Input: part model. Units: mm. Frame: model coordinates. A direction names the side the tool comes from. Round coordinates to 2 decimals unless told otherwise and drop trailing zeros. Loops run counter-clockwise (first coordinate to the right, second up) from the corner with the lowest first, then second, coordinate; pieces in that order, holes last. Notation, with made-up numbers: M -16.75,-3 L 31.25,-3 A19 ccw 31.25,16 Z; hole C 11,-28.5 d3. An arc over 180 degrees is marked long. Return JSON: item names as keys, results as strings. Group by question number.
1) Section D-D (z = 24). Output: boundary loops of the cut face in (x, y), plus the area to 3 significant figures.
2) Mould query, pull axis X, two halves, no side actions, for faces 1 (the face through (-34.962, 11.959, -7.764)), 2 (the face through (-7.5, 0, -8.5)), 3 (the face through (-3.3, 3.73, 10.48)). Classes: +X half, -X half, draft (parallel to the pull), parting line (faces both ways), or undercut.
3) Section A-A (z = 0). Output: boundary loops of the cut face in (x, y).
4) Section B-B (x = 0). Output: boundary loops of the cut face in (y, z), plus the area to 3 significant figures.
5) Section C-C (y = 11.5). Output: boundary loops of the cut face in (x, z).
6) Access query for faces 4 (the face through (3.3, 20.63, 10.48)), 5 (the face through (-9.21, 12.2, -2.05)), 6 (the face through (-9, 7.353, -3.31)). Directions: +Z, -Z, +X, -X, +Y, -Y. A direction counts if a zero-diameter tool reaches every point of the face in a straight line with its end or side. Return the directions, or none.
7) Contact query for flat-ended pins moving along their axis: P1, Ø12, axis at y = 18, z = 11.5, coming from the +X side; P2, Ø10, axis at x = 19.5, y = 19, coming from the +Z side; P3, Ø10, axis at y = 19, z = -13.5, coming from the +X side; P4, Ø13, axis at x = 0, z = 0, coming from the -Y side. Output: stop coordinate, or through.
8) Material intervals for line 1 (X direction, y = 3.5, z = 0); line 2 (X direction, y = 13.25, z = 0); line 3 (Z direction, x = -2.5, y = 15), sorted ascending. Write a range as from..to.
from build123d import *

# Parameters (mm, degrees)
SKETCH1_R           = 35.814
BOSS_EXTRUDE1_DEPTH = 24.257
SKETCH2_R           = 9.4361
CUT_EXTRUDE1_DEPTH  = 57.157699748
SKETCH3_R           = 10.9855
CUT_EXTRUDE2_DEPTH  = 7.3533
CUT_EXTRUDE3_START  = -7.3533
SKETCH4_R           = 10.9855
CUT_EXTRUDE3_DEPTH  = 7.3533


with BuildPart() as part:
    # Sketch1 → Boss-Extrude1 (new body)
    with BuildSketch(Plane(origin=(0, 0, 0), x_dir=(1, 0, 0), z_dir=(0, 1, 0))):
        with Locations(Location((0, 0, 0), (0, 0, 270))):
            Circle(SKETCH1_R)
    extrude(amount=BOSS_EXTRUDE1_DEPTH)

    # Sketch2 → Cut-Extrude1 (cut, through all)
    with BuildSketch(Plane(origin=(0, 24.257, 0), x_dir=(1, 0, 0), z_dir=(0, 1, 0))):
        with Locations(Location((0, 0, 0), (0, 0, 270))):
            Circle(SKETCH2_R)
    extrude(amount=-CUT_EXTRUDE1_DEPTH, mode=Mode.SUBTRACT)

    # Sketch3 → Cut-Extrude2 (cut)
    with BuildSketch(Plane(origin=(0, 24.257, 0), x_dir=(1, 0, 0), z_dir=(0, 1, 0))):
        with Locations(Location((0, 0, 0), (0, 0, 270))):
            Circle(SKETCH3_R)
    extrude(amount=-CUT_EXTRUDE2_DEPTH, mode=Mode.SUBTRACT)

    # Sketch4 → Cut-Extrude3 (cut)
    with BuildSketch(Plane.XZ.offset(CUT_EXTRUDE3_START)):
        with Locations(Location((0, 0, 0), (0, 0, 90))):
            Circle(SKETCH4_R)
    extrude(amount=CUT_EXTRUDE3_DEPTH, mode=Mode.SUBTRACT)


solid = part.part
Returned:
{
 "1": {"outline": "M -26.58,0 L 26.58,0 L 26.58,24.26 L -26.58,24.26 Z", "area": "1,290 mm^2"},
 "2": {"face 1": "parting line", "face 2": "draft", "face 3": "undercut"},
 "3": {"outline": "M -35.81,0 L -10.99,0 L -10.99,7.35 L -9.44,7.35 L -9.44,16.9 L -10.99,16.9 L -10.99,24.26 L -35.81,24.26 Z; M 9.44,7.35 L 10.99,7.35 L 10.99,0 L 35.81,0 L 35.81,24.26 L 10.99,24.26 L 10.99,16.9 L 9.44,16.9 Z"},
 "4": {"outline": "M 0,-35.81 L 24.26,-35.81 L 24.26,-10.99 L 16.9,-10.99 L 16.9,-9.44 L 7.35,-9.44 L 7.35,-10.99 L 0,-10.99 Z; M 0,10.99 L 7.35,10.99 L 7.35,9.44 L 16.9,9.44 L 16.9,10.99 L 24.26,10.99 L 24.26,35.81 L 0,35.81 Z", "area": "1,230 mm^2"},
 "5": {"outline": "C 0,0 d71.63; hole C 0,0 d18.87"},
 "6": {"face 4": "+Y", "face 5": "+Y, -Y", "face 6": "-Y"},
 "7": {"P1": "stops at x = 35.39", "P2": "stops at z = 32.75", "P3": "stops at x = 34.79", "P4": "passes through"},
 "8": {"line 1": "x = -35.81..-10.99, 10.99..35.81", "line 2": "x = -35.81..-9.44, 9.44..35.81", "line 3": "z = -35.73..-9.1, 9.1..35.73"}
}
